from build123d import *

# Parameters (mm, degrees)
IZIM2_W                     = 2
IZIM2_H                     = 0.3
KES_EKSTR_ZYON3_DEPTH       = 10
IZIM3_W                     = 0.6
IZIM3_H                     = 0.6
Y_KSEKLIK_EKSTR_ZYON1_DEPTH = 2.75
IZIM4_W                     = 0.6
IZIM4_H                     = 0.6
Y_KSEKLIK_EKSTR_ZYON2_DEPTH = 4.36
RADYUS1_R                   = 0.5
RADYUS2_R                   = 0.15
RADYUS3_R                   = 0.15


with BuildPart() as part:
    # Çizim1 → Döndür1 (revolve)
    with BuildSketch(Plane.XY, mode=Mode.PRIVATE) as d_nd_r1_sk:
        with BuildLine():
            Line((2.357986429, 1), (2.357986429, 7.01))
            ThreePointArc((2.357986429, 7.01), (1.450534384, 8.233870055), (0, 8.7))
            Line((0, 8.7), (0, 1))
            Line((0, 1), (2.357986429, 1))
        make_face()
        Polygon((2.657986429, 1), (2.357986429, 1), (0, 1), (0, 0), (2.657986429, 0), align=None)
    revolve(d_nd_r1_sk.sketch.rotate(Axis((0, 8.7, 0), (0, -1, 0)), 180), axis=Axis((0, 8.7, 0), (0, -1, 0)))

    # Çizim2 → Kes-Ekstrüzyon3 (cut)
    with BuildSketch(Plane(origin=(0, 0, 0), x_dir=(-1, 0, 0), z_dir=(0, -1, 0))):
        with Locations((-0.070058143, -2.64)):
            Rectangle(IZIM2_W, IZIM2_H)
    extrude(amount=-KES_EKSTR_ZYON3_DEPTH, mode=Mode.SUBTRACT)

    # Çizim3 → Yükseklik-Ekstrüzyon1 (add)
    with BuildSketch(Plane.XZ):
        with Locations((0, 1.27)):
            Rectangle(IZIM3_W, IZIM3_H)
        with Locations((0, -1.27)):
            Rectangle(IZIM3_W, IZIM3_H)
    extrude(amount=Y_KSEKLIK_EKSTR_ZYON1_DEPTH)

    # Çizim4 → Yükseklik-Ekstrüzyon2 (add)
    with BuildSketch(Plane(origin=(0.3, 0, 0), x_dir=(0, 0, -1), z_dir=(1, 0, 0))):
        with Locations((-1.27, -2.45)):
            Rectangle(IZIM4_W, IZIM4_H)
        with Locations((1.27, -2.45)):
            Rectangle(IZIM4_W, IZIM4_H)
    extrude(amount=Y_KSEKLIK_EKSTR_ZYON2_DEPTH)

    # Radyus1
    radyus1_edges = [part.edges().sort_by_distance(p)[0] for p in [
        (-0.3, -2.75, 1.27),
        (-0.3, -2.75, -1.27),
    ]]
    fillet(radyus1_edges, radius=RADYUS1_R)

    # Radyus2
    radyus2_edges = [part.edges().sort_by_distance(p)[0] for p in [
        (0.3, -2.15, -1.27),
    ]]
    fillet(radyus2_edges, radius=RADYUS2_R)

    # Radyus3
    radyus3_edges = [part.edges().sort_by_distance(p)[0] for p in [
        (0.3, -2.15, 1.27),
    ]]
    fillet(radyus3_edges, radius=RADYUS3_R)


solid = part.part
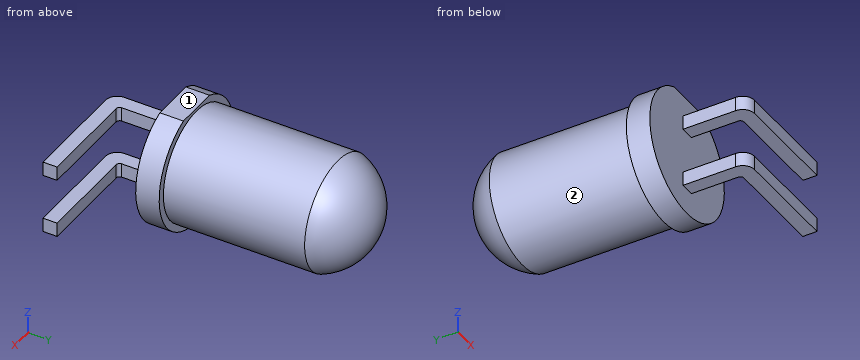
Input: part model. Units: mm. Frame: model coordinates. Face numbers are marked on the shaded views. A direction names the side the tool comes from. Coordinates: 2 decimals unless noted, no trailing zeros. Loops run counter-clockwise (first coordinate to the right, second up) from the corner with the lowest first, then second, coordinate; pieces in that order, holes last.
Q1. Cut plane D-D (x = 1.25). Output: boundary loops of the cut face in (y, z).
Q2. Material intervals for line 1 (Z direction, x = 0, y = -0.5); line 2 (Y direction, x = -2, z = 1.5); line 3 (Y direction, x = 3.25, z = 1.45), sorted ascending.
Q3. Cut plane A-A (y = -1.25). Output: boundary loops of the cut face in (x, z), then the cut area to 3 significant figures.
Q4. Cut plane B-B (x = 3.5). Output: boundary loops of the cut face in (y, z), then the cut area to 3 significant figures.
Q5. Cut plane C-C (z = 0). Output: boundary loops of the cut face in (x, y).
Q6. Contact query for flat-ended pins moving along their axis: pin 1 (0.8 mm diameter, centred on x = 3, y = -2, fed in from -Z); pin 2 (0.5 mm diameter, centred on x = 3.5, z = 1.5, fed in from +Y); pin 3 (0.5 mm diameter, centred on y = -1, z = 1.5, fed in from +X). Output: stop coordinate, or through.
Q7. Set-up query: the marked faces 1 and 2. Return all of +Z, -Z, +X, -X, +Y, -Y with unobstructed straight access to the full face (end or side cutting, diameter ignored); none if empty.
Working result:
1. outline: (-2.75, -1.57) - (-2.15, -1.57) - (-2.15, -0.97) - (-2.75, -0.97) - close; (-2.75, 0.97) - (-2.15, 0.97) - (-2.15, 1.57) - (-2.75, 1.57) - close; (0, -2.35) - (1, -2.35) - (1, -2) - (7.01, -2) arc R2.15 ccw to (7.01, 2) - (1, 2) - (1, 2.35) - (0, 2.35) - close
2. line 1: z = -1.57 to -0.97, 0.97 to 1.57
2. line 2: y = 0 to 1
2. line 3: y = -2.75 to -2.15
3. outline: (-0.3, -1.57) - (0.3, -1.57) - (0.3, -0.97) - (-0.3, -0.97) - close; (-0.3, 0.97) - (0.3, 0.97) - (0.3, 1.57) - (-0.3, 1.57) - close
3. area: 0.720 mm2
4. outline: (-2.75, -1.57) - (-2.15, -1.57) - (-2.15, -0.97) - (-2.75, -0.97) - close; (-2.75, 0.97) - (-2.15, 0.97) - (-2.15, 1.57) - (-2.75, 1.57) - close
4. area: 0.720 mm2
5. outline: (-2.66, 0) - (2.66, 0) - (2.66, 1) - (2.36, 1) - (2.36, 7.01) arc R2.49 ccw to (-2.36, 7.01) - (-2.36, 1) - (-2.66, 1) - close
6. pin 1: stops at z = -1.57
6. pin 2: stops at y = -2.15
6. pin 3: stops at x = 0.3
7. face 1: +Z, +X, -X, +Y, -Y
7. face 2: +Y
